Here's the drawing with two shaded views (mm, measured from the low corner). I have some questions. A direction names the side the tool comes from. Coordinates: 2 decimals unless noted, no trailing zeros. Write each loop counter-clockwise with the first axis right and the second up, starting at its lowest first coordinate (ties: lowest second). Pieces come first, ordered by that corner, then holes.
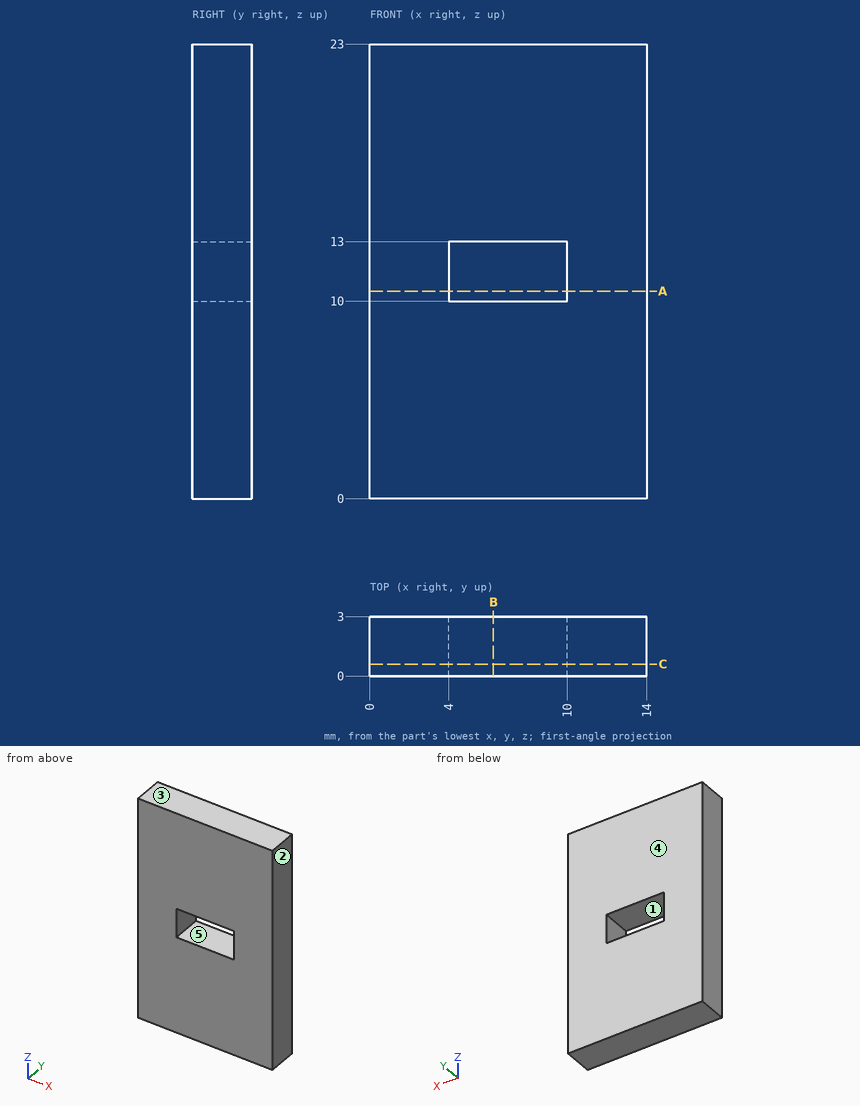
1. If we section it at C-C, the plane y = 0.6: List the corners of the cut face in (x, z) for me, plus the area to 3 significant figures.
2. If we section it at A-A, the plane z = 10.5: List the corners of the cut face in (x, y) for me.
3. If we section it at B-B, the plane x = 6.25: List the corners of the cut face in (y, z) for me, plus the area to 3 significant figures.
4. We'd pull the mould along X, two halves only. Please class the marked faces 1, 2 and 3: released by +X, released by -X, zero draft, split by the parting line, or undercut.
5. Which directions (+Z, -Z, +X, -X, +Y, -Y) give clear straight access to the entire face, cutting with the end or side of a thin tool? Please do the marked faces 4 and 5.
6. If I drill on L1, parallel to Z at x = 5.5, y = 0.9, over which ranges is the centre line in solid material (lowest first)?
Answers:
1. outline: (0, 0) - (14, 0) - (14, 23) - (0, 23) - close; hole (4, 10) - (10, 10) - (10, 13) - (4, 13) - close
1. area: 304 mm2
2. outline: (0, 0) - (4, 0) - (4, 3) - (0, 3) - close; (10, 0) - (14, 0) - (14, 3) - (10, 3) - close
3. outline: (0, 0) - (3, 0) - (3, 10) - (0, 10) - close; (0, 13) - (3, 13) - (3, 23) - (0, 23) - close
3. area: 60.0 mm2
4. face 1: undercut
4. face 2: released by +X
4. face 3: zero draft
5. face 4: +Z, -Z, +X, -X, +Y
5. face 5: +Y, -Y
6. L1: z = 0 to 10, 13 to 23
